CAD build for the part. Positions are in the model's coordinates, mm. A direction names the side the tool comes from. Round coordinates to 2 decimals unless told otherwise and drop trailing zeros. Order: outer loops, then holes, each group sorted by start corner. A loop starts at its lowest first (then second) coordinate and runs counter-clockwise, first axis right, second up.
```python
from build123d import *

# Parameters (mm, degrees)
SKETCH1_R           = 10
BOSS_EXTRUDE1_DEPTH = 25
SKETCH2_W           = 0.8
SKETCH2_H           = 5
BOSS_EXTRUDE2_DEPTH = 8
BOSS_EXTRUDE3_DEPTH = 1.2
SKETCH4_W           = 17
SKETCH4_H           = 7
CUT_EXTRUDE1_DEPTH  = 6
SKETCH5_W           = 2
SKETCH5_H           = 7
CUT_EXTRUDE2_DEPTH  = 4
CUT_EXTRUDE3_DEPTH  = 25
SKETCH7_W           = 5
SKETCH7_H           = 8
BOSS_EXTRUDE4_DEPTH = 0.8
CUT_EXTRUDE4_REACH  = 29.409


with BuildPart() as part:
    # Sketch1 → Boss-Extrude1 (new body)
    with BuildSketch(Plane(origin=(0, 0, 0), x_dir=(1, 0, 0), z_dir=(0, 1, 0))):
        with Locations(Location((0, 0, 0), (0, 0, 270))):
            Circle(SKETCH1_R)
    extrude(amount=BOSS_EXTRUDE1_DEPTH)

    # Sketch4 → Cut-Extrude1 (cut)
    with BuildSketch(Plane(origin=(0, 25, 0), x_dir=(1, 0, 0), z_dir=(0, 1, 0))):
        Rectangle(SKETCH4_W, SKETCH4_H)
    extrude(amount=-CUT_EXTRUDE1_DEPTH, mode=Mode.SUBTRACT)

    # Sketch5 → Cut-Extrude2 (cut)
    with BuildSketch(Plane(origin=(0, 19, 0), x_dir=(1, 0, 0), z_dir=(0, 1, 0))):
        with Locations((-2.25, 0)):
            Rectangle(SKETCH5_W, SKETCH5_H)
    extrude(amount=-CUT_EXTRUDE2_DEPTH, mode=Mode.SUBTRACT)

    # Sketch6 → Cut-Extrude3 (cut)
    with BuildSketch(Plane.XZ):
        with BuildLine():
            Line((-8.644632716, 5.026959838), (8.644632716, 5.026959838))
            ThreePointArc((8.644632716, 5.026959838), (0, 10), (-8.644632716, 5.026959838))
        make_face()
        with BuildLine():
            Line((-8.644632716, -5.026959838), (8.644632716, -5.026959838))
            ThreePointArc((8.644632716, -5.026959838), (0, -10), (-8.644632716, -5.026959838))
        make_face()
    extrude(amount=-CUT_EXTRUDE3_DEPTH, mode=Mode.SUBTRACT)



with BuildPart() as body_2:
    # Sketch2 → Boss-Extrude2 (new body)
    with BuildSketch(Plane(origin=(0, 0, 0), x_dir=(-1, 0, 0), z_dir=(0, -1, 0))):
        with Locations((7.65, 0)):
            Rectangle(SKETCH2_W, SKETCH2_H)
    extrude(amount=BOSS_EXTRUDE2_DEPTH)

    # Sketch3 → Boss-Extrude3 (add)
    with BuildSketch(Plane.ZY.offset(8.05)):
        Polygon((-2.5, -8), (-2.5, 0), (2.5, 0), (2.5, -8), (1.5, -8), (1.5, -0.75), (-1.5, -0.75), (-1.5, -8), align=None)
    extrude(amount=BOSS_EXTRUDE3_DEPTH)


with BuildPart() as part_1:
    add(part.part)

    add(body_2.part)  # Boss-Extrude4 merges body 2
    # Sketch7 → Boss-Extrude4 (add)
    with BuildSketch(Plane.ZY.offset(9.25)):
        with Locations((0, -4)):
            Rectangle(SKETCH7_W, SKETCH7_H)
    extrude(amount=BOSS_EXTRUDE4_DEPTH)

    # Sketch8 → Cut-Extrude4 (cut, up to next)
    with BuildSketch(Plane(origin=(0, 0, 0), x_dir=(1, 0, 0), z_dir=(0, 1, 0)), mode=Mode.PRIVATE) as cut_extrude4_sk1:
        with BuildLine():
            Line((-9.682458366, 2.5), (-10.05, 2.5))
            Line((-10.05, 2.5), (-10.05, -2.5))
            Line((-10.05, -2.5), (-9.682458366, -2.5))
            ThreePointArc((-9.682458366, -2.5), (-10, 0), (-9.682458366, 2.5))
        make_face()
    cut_extrude4_tool1 = extrude(cut_extrude4_sk1.sketch, amount=-CUT_EXTRUDE4_REACH, mode=Mode.PRIVATE) & part_1.part
    add(cut_extrude4_tool1.solids().sort_by_distance((-9.866229, 0, -2.449865))[0], mode=Mode.SUBTRACT)


solid = part_1.part
```
1. Cut at B-B, the plane z = -2. Write the cut outline in (x, y), and give its area (3 significant figures).
2. Pin check, flat tips, straight feed: P1, Ø1.9, axis at x = -8.5, y = -3.5, coming from the -Z side; P2, Ø1, axis at x = 0.5, z = 0.5, coming from the +Y side; P3, Ø1.9, axis at x = -8.5, y = -4, coming from the +Z side. Stop position of each tip, or through.
3. Cut at A-A, the plane x = 3. Write the cut outline in (y, z).
4. Mould opens along X. For faces 6 (the face through (0, 22, 3.5)), 7 (the face through (-3.25, 17, 0)), 8 (the face through (0, 25, 4)), 9 (the face through (10, 12, 0)) say: released by +X, released by -X, zero draft, split by the parting line, or undercut.
5. Cut at C-C, the plane y = 12.5. Write the cut outline in (x, z), and give its area (3 significant figures).
6. Drill centre lines: line 1 (Z direction, x = 0.5, y = 21.5); line 2 (Z direction, x = -9, y = -2); line 3 (Y direction, x = -6.5, z = -1.25). Where is each one in solid material? Low to high.
7. Cut at D-D, the plane z = 0.25. Write the cut outline in (x, y), and give its area (3 significant figures).
8. Tool access for faces 1 (the face through (-8, -4, 2.5)), 2 (the face through (-1.25, 17, 0)), 3 (the face through (-9.25, -4, 0)), 4 (the face through (-8, -4, -2.5)), 5 (the face through (-7.25, -4, 0)): list every direction of +Z, -Z, +X, -X, +Y, -Y with a clear straight run to the whole face (end or side of a thin tool).
Outcome:
1. outline: (-9.8, -8) - (-7.25, -8) - (-7.25, 0) - (9.8, 0) - (9.8, 25) - (8.5, 25) - (8.5, 19) - (-1.25, 19) - (-1.25, 15) - (-3.25, 15) - (-3.25, 19) - (-8.5, 19) - (-8.5, 25) - (-9.8, 25) - close
1. area: 400 mm2
2. P1: stops at z = -2.5
2. P2: stops at y = 19
2. P3: stops at z = 2.5
3. outline: (0, -5.03) - (25, -5.03) - (25, -3.5) - (19, -3.5) - (19, 3.5) - (25, 3.5) - (25, 5.03) - (0, 5.03) - close
4. face 6: undercut
4. face 7: undercut
4. face 8: zero draft
4. face 9: released by +X
5. outline: (-8.64, -5.03) - (8.64, -5.03) arc R10 ccw to (8.64, 5.03) - (-8.64, 5.03) arc R10 ccw to start
5. area: 192 mm2
6. line 1: z = -5.03 to -3.5, 3.5 to 5.03
6. line 2: z = -2.5 to -1.5, 1.5 to 2.5
6. line 3: y = 0 to 19
7. outline: (-10, -8) - (-9.25, -8) - (-9.25, -0.75) - (-8.05, -0.75) - (-8.05, -8) - (-7.25, -8) - (-7.25, 0) - (10, 0) - (10, 25) - (8.5, 25) - (8.5, 19) - (-1.25, 19) - (-1.25, 15) - (-3.25, 15) - (-3.25, 19) - (-8.5, 19) - (-8.5, 25) - (-10, 25) - close
7. area: 403 mm2
8. face 1: +Z, +X, -X, -Y
8. face 2: +Y
8. face 3: -Y
8. face 4: -Z, +X, -X, -Y
8. face 5: +Z, -Z, +X, -Y
